Build history of the part. All positions in model axes, mm. A direction names the side the tool comes from. Round coordinates to 2 decimals unless told otherwise and drop trailing zeros. Write each loop counter-clockwise with the first axis right and the second up, starting at its lowest first coordinate (ties: lowest second). Pieces come first, ordered by that corner, then holes. Notation, with made-up numbers: M 22.5,78 L 36.5,78 A31 ccw 36.5,103 Z; hole C -1.75,19.5 d5. An arc over 180 degrees is marked long. Write item = value, one per line. Start each with the question number.
Q1. Drop flat-ended pins along their axis: P1, Ø2, axis at x = 66, y = -2, coming from the -Z side; P2, Ø1.5, axis at x = 33.5, y = -2, coming from the +Z side. Give the stop position or say it passes through.
Q2. Band-saw the part on B-B on x = 58.5. Write the cut outline in (y, z).
Q3. Tool access for faces 3 (the cylindrical face through (45.908, -0.165, -33.746)), 4 (the flat face through (0, 0, 0)), 5 (the cylindrical face through (93.8, 2.28, -9.86)): list every direction of +Z, -Z, +X, -X, +Y, -Y with a clear straight run to the whole face (end or side of a thin tool).
Q4. Band-saw the part on A-A on y = 0. Write the cut outline in (x, z).
Q5. Probe L1, parallel to X at y = 1.75, z = -2; L2, parallel to Z at x = 56.5, y = 0.25; L3, parallel to X at y = 2.25, z = -23. List the from-to ranges inside material, lowest first.
Q6. Pull direction X, two halves, no side cores. Call faces 1 (the flat face through (91, 0, 0)), 2 (the cylindrical face through (-3.746, -0.165, -10.14)): released by +X, released by -X, zero draft, split by the parting line, or undercut.
```python
from build123d import *

# Parameters (mm, degrees)
CROQUIS2_R = 3.75


with BuildPart() as part:
    # Barrer1: sweep along a path in Croquis1
    with BuildLine(Plane(origin=(0, 0, 0), x_dir=(1, 0, 0), z_dir=(0, 1, 0))) as barrer1_path:
        Line((0, 0), (0, 20))
        ThreePointArc((0, 20), (2.928932188, 27.071067812), (10, 30))
        Line((10, 30), (80.824, 30))
        ThreePointArc((80.824, 30), (87.895067812, 27.071067812), (90.824, 20))
        Line((90.824, 20), (90.824, 0))
    # Croquis2 → Barrer1 (sweep)
    with BuildSketch(Plane.XY):
        Circle(CROQUIS2_R)
    sweep(path=barrer1_path.line)


solid = part.part
```
Conclusion:
q1.P1 = -33.61
q1.P2 = -26.46
q2.outline = C 0,-30 d7.5
q3.face_3 = none
q3.face_4 = +Z, +X, -X, +Y, -Y
q3.face_5 = +Z
q4.outline = M -3.75,-20 A13.75 ccw 10,-33.75 L 80.82,-33.75 A13.75 ccw 94.57,-20 L 94.57,0 L 87.07,0 L 87.07,-20 A6.25 cw 80.82,-26.25 L 10,-26.25 A6.25 cw 3.75,-20 L 3.75,0 L -3.75,0 Z
q5.L1 = -3.32 to 3.32, 87.51 to 94.14
q5.L2 = -33.74 to -26.26
q5.L3 = -2.65 to 3.68, 87.15 to 93.47
q6.face_1 = zero draft
q6.face_2 = undercut
